from build123d import *

# Parameters (mm, degrees)
SKETCH1_R      = 63.5
EXTRUDE1_DEPTH = 1.95
SKETCH2_R      = 51
EXTRUDE2_DEPTH = 4
SKETCH3_R      = 50
EXTRUDE3_DEPTH = 91.158194303
SKETCH5_R      = 2.54


with BuildPart() as part:
    # Sketch1 → Extrude1 (new, symmetric)
    with BuildSketch(Plane.XY):
        Circle(SKETCH1_R)
    extrude(amount=EXTRUDE1_DEPTH, both=True)

    # Sketch2 → Extrude2 (add, symmetric)
    with BuildSketch(Plane.XY):
        Circle(SKETCH2_R)
    extrude(amount=EXTRUDE2_DEPTH, both=True)

    # Sketch3 → Extrude3 (cut, through all)
    with BuildSketch(Plane.XY.offset(4)):
        Circle(SKETCH3_R)
    extrude(amount=-EXTRUDE3_DEPTH, mode=Mode.SUBTRACT)

    # Sketch5 → Revolve2 (revolve)
    with BuildSketch(Plane(origin=(0, 0, 0), x_dir=(0, 0, -1), z_dir=(1, 0, 0)), mode=Mode.PRIVATE) as revolve2_sk:
        with Locations((0, 54.54)):
            Circle(SKETCH5_R)
    revolve(revolve2_sk.sketch.rotate(Axis((0, 0, 4), (0, 0, -1)), 90), axis=Axis((0, 0, 4), (0, 0, -1)))

    # Sketch6 → Cut-Revolve1 (revolve, cut)
    with BuildSketch(Plane(origin=(0, 0, 0), x_dir=(0, 0, -1), z_dir=(1, 0, 0)), mode=Mode.PRIVATE) as cut_revolve1_sk:
        with BuildLine():
            Line((-1, 63.5), (-1, 62))
            ThreePointArc((-1, 62), (0, 61), (1, 62))
            Line((1, 62), (1, 63.5))
            Line((1, 63.5), (-1, 63.5))
        make_face()
    revolve(cut_revolve1_sk.sketch.rotate(Axis((0, 0, 4), (0, 0, -1)), 180), axis=Axis((0, 0, 4), (0, 0, -1)), mode=Mode.SUBTRACT)


solid = part.part
The listing builds one solid part. Answer for the finished solid, in the listing's coordinates (mm). A direction names the side the tool comes from. Give positions to 0.01 mm unless a question says otherwise; leave off trailing zeros. Answer as a JSON object with one key per item and string values.
1. For faces 5 (the flat face through (4.41, -56.15, -1.95)), 6 (the flat face through (4.41, -56.15, 1.95)), 7 (the flat face through (33.8, -37.5, -4)), determine the directions among +Z, -Z, +X, -X, +Y, -Y from which every point of the face is accessible in a straight line to the end or side of a thin tool.
Determined:
{"face 5": "-Z", "face 6": "+Z", "face 7": "-Z, +X, -X, +Y, -Y"}
2. Find the intervals of material crossed by L1, parallel to Z at x = 22, y = 58.5; L2, parallel to Y at x = 0, z = 1.75; L3, parallel to X at y = 19, z = 1.5, in increasing order. Write a range as [from, to].
Determined:
{"L1": "[-1.95, -1], [1, 1.95]", "L2": "[-63.5, -50], [50, 63.5]", "L3": "[-60.59, -46.25], [46.25, 60.59]"}
3. Flat-ended cylindrical pins translate along their axes: pin 1 Ø3 at (y, z) = (-17, 3) entering from -X; pin 2 Ø1 at (x, z) = (49, 1.5) entering from +Y; pin 3 Ø2 at (x, z) = (-1, 1.5) entering from -Y. Find the tip coordinate at first contact, or state that the pin passes through.
Determined:
{"pin 1": "x = -61.47", "pin 2": "y = 40.99", "pin 3": "y = -63.5"}
4. For a pull along Z with two mould halves and no side action, classify faces 1 (the flat face through (61, -14, 1)), 2 (the flat face through (-28, 43, -1.95)), 3 (the flat face through (14, 61, -1)), 4 (the cylindrical face through (60.57, 19.07, -1.47)) as pulls with the +Z half, pulls with the -Z half, needs draft (parallel to the pull), parting line crosses it, or undercut.
Determined:
{"face 1": "undercut", "face 2": "pulls with the -Z half", "face 3": "undercut", "face 4": "needs draft"}
